The figure shows three views and two pictorial views of one solid part (mm, origin at its lowest corner). Answer the questions. A direction names the side the tool comes from. Round coordinates to 2 decimals unless told otherwise and drop trailing zeros. Order: outer loops, then holes, each group sorted by start corner. A loop starts at its lowest first (then second) coordinate and runs counter-clockwise, first axis right, second up. Notation, with made-up numbers: (-33.75, -40) -> (18.25, -40) arc R10 ccw to (18.25, -29) -> close; hole circle Ø10 at (60, -1). An arc over 180 degrees is marked (long way). Answer as a JSON object with one key per item and string values. Group by question number.
Item 1: Section B-B, the plane x = 8.5 is taken. Write down the section's boundary in (y, z) (1 decimal).
Item 2: Section C-C, the plane x = 21 is taken. Write down the section's boundary in (y, z) (1 decimal), plus the area to 3 significant figures.
Item 3: Section A-A, the plane z = 5.5 is taken. Write down the section's boundary in (x, y).
Item 4: Consider probe 1 along X at (y, z) = (1.05, 5.5); probe 2 along X at (y, z) = (2.5, 6); probe 3 along X at (y, z) = (8.25, 13.5). Determine where each line is inside the solid, lowest interval first. Write a range as from..to.
Item 5: The mould has two halves that part along Y. Classify the marked faces 4, 5, 6 and 7: pulls with the +Y half, pulls with the -Y half, needs draft (parallel to the pull), parting line crosses it, or undercut.
Item 6: For the marked faces 1, 2 and 3, determine the directions among +Z, -Z, +X, -X, +Y, -Y from which every point of the face is accessible in a straight line to the end or side of a thin tool.
Item 7: Given P1, Ø3, axis at y = 15, z = 18, coming from the +X side; P2, Ø9, axis at x = 21, z = 6, coming from the +Y side (1 decimal); P3, Ø1, axis at y = 5, z = 9, coming from the +X side; P4, Ø6.5, axis at x = 5.5, z = 5.5, coming from the +Y side, each flat-ended and moving along its own axis, determine where each tip first touches the part or whether it passes through.
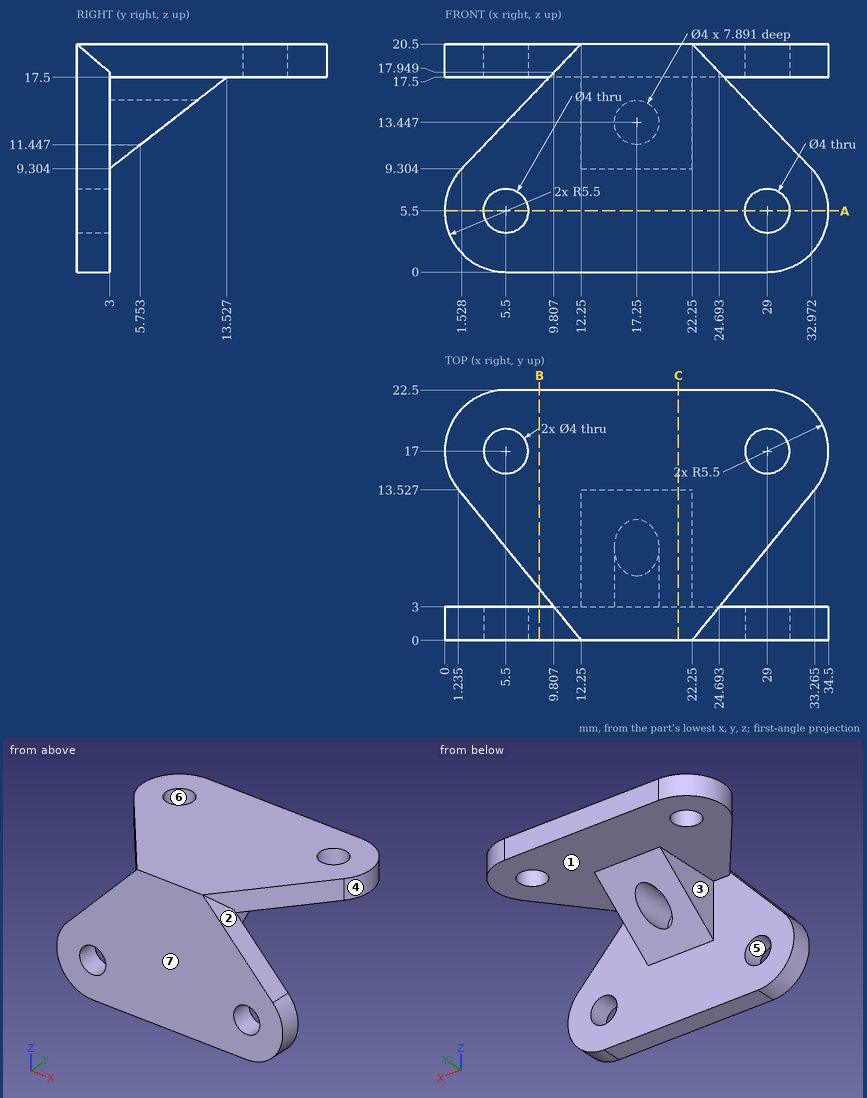
Values found:
{
 "1": {"outline": "(0, 0) -> (3, 0) -> (3, 16.6) -> (0, 16.6) -> close; (4.6, 17.5) -> (22.5, 17.5) -> (22.5, 20.5) -> (4.6, 20.5) -> close"},
 "2": {"outline": "(0, 0) -> (3, 0) -> (3, 9.3) -> (13.5, 17.5) -> (22.5, 17.5) -> (22.5, 20.5) -> (0, 20.5) -> close", "area": "163 mm2"},
 "3": {"outline": "(0, 0) -> (3.5, 0) -> (3.5, 3) -> (0, 3) -> close; (7.5, 0) -> (27, 0) -> (27, 3) -> (7.5, 3) -> close; (31, 0) -> (34.5, 0) -> (34.5, 3) -> (31, 3) -> close"},
 "4": {"probe 1": "0..3.5, 7.5..27, 31..34.5", "probe 2": "0.02..3.56, 7.44..27.06, 30.94..34.48", "probe 3": "12.25..15.25, 19.25..22.25"},
 "5": {"face 4": "parting line crosses it", "face 5": "needs draft", "face 6": "undercut", "face 7": "pulls with the -Y half"},
 "6": {"face 1": "-Z, +Y", "face 2": "+Z, +X, -Y", "face 3": "-Z, -X, +Y"},
 "7": {"P1": "x = 34.48", "P2": "y = 4.5", "P3": "through", "P4": "y = 3"}
}
